from build123d import *

# Parameters (mm, degrees)
BOSS_EXTRUDE1_DEPTH      = 2.5
SKETCH1_R                = 3.11925
SKETCH1_R_2              = 1.61925
BOSS_EXTRUDE2_DEPTH      = 2.5
SKETCH12_R               = 1.61925
CUT_EXTRUDE2_DEPTH       = 3.5
SKETCH15_R               = 3
BOSS_EXTRUDE6_DEPTH      = 2.5
SKETCH13_R               = 1.5
CUT_EXTRUDE5_DEPTH       = 3.5
CUT_EXTRUDE5_DEPTH_BACK  = 3.5
SKETCH16_R               = 3.25
SKETCH16_R_2             = 3.255054338
BOSS_EXTRUDE7_DEPTH      = 2.5
SKETCH17_R               = 1.75
SKETCH17_R_2             = 1.755054338
CUT_EXTRUDE6_DEPTH       = 1
CUT_EXTRUDE6_DEPTH_BACK  = 6
SKETCH24_R               = 1.534588162
SKETCH24_R_2             = 1.539679215
SKETCH24_R_3             = 1.53510928
SKETCH24_R_4             = 1.507254119
SKETCH24_R_5             = 1.501766116
SKETCH24_R_6             = 1.506723366
CUT_EXTRUDE7_DEPTH       = 3.5
CUT_EXTRUDE7_DEPTH_BACK  = 3.5
BOSS_EXTRUDE8_DEPTH      = 23
SKETCH28_W               = 1.910572049
SKETCH28_H               = 15
SKETCH28_W_2             = 2.161085764
CUT_EXTRUDE9_DEPTH       = 3.5
SKETCH30_W               = 30
SKETCH30_H               = 12
SKETCH30_W_2             = 8.543214141
SKETCH30_H_2             = 45.874985667
SKETCH30_H_3             = 29.216310988
SKETCH30_W_3             = 26.664834195
SKETCH30_H_4             = 26.922465443
SKETCH30_W_4             = 17.818641616
SKETCH30_H_5             = 15.402052611
SKETCH30_W_5             = 8.591934673
SKETCH30_H_6             = 73.671406809
CUT_EXTRUDE11_DEPTH      = 3.5
SKETCH29_R               = 12.3
CUT_EXTRUDE12_DEPTH      = 66.426944419
CUT_EXTRUDE12_DEPTH_BACK = 50.584496916
SKETCH31_R               = 1.5
CUT_EXTRUDE13_DEPTH      = 19.369261936
CUT_EXTRUDE13_DEPTH_BACK = 3.5
CUT_EXTRUDE14_DEPTH      = 12


with BuildPart() as part:
    # Sketch2 → Boss-Extrude1 (new body)
    with BuildSketch(Plane(origin=(0, -17.332299444, 0), x_dir=(-1, 0, 0), z_dir=(0, -1, 0))):
        Polygon((125.241603418, -58.531029956), (125.241603418, 41.468970044), (125.241603418, 48.975336237), (115.668802349, 48.975336237), (115.668802349, 41.468970044), (53.135946408, 41.468970044), (53.135946408, 48.975336237), (43.168799778, 48.975336237), (43.168799778, 41.468970044), (-19.254443916, 41.468970044), (-19.254443916, 48.975336237), (-29.674557938, 48.975336237), (-29.674557938, 41.234228149), (-53.610322333, 9.147791006), (-53.610322333, -26.975248892), (-29.352965282, -57.102703243), (-29.352965282, -66.036105098), (-19.352967368, -66.036105098), (-19.352967368, -58.531029956), (43.147035426, -58.531029956), (43.147035426, -66.036105098), (53.147035202, -66.036105098), (53.147035202, -58.531029956), (115.647037996, -58.531029956), (115.647037996, -66.036105098), (125.241603418, -66.036105098), align=None)
    extrude(amount=-BOSS_EXTRUDE1_DEPTH)

    # Sketch1 → Boss-Extrude2 (add)
    with BuildSketch(Plane(origin=(-134.962394185, -12.332299444, 36.871029956), x_dir=(1, 0, 0), z_dir=(0, 1, 0))):
        with Locations((14.01445, 2.71145)):
            Circle(SKETCH1_R)
        with Locations((14.01445, 2.71145)):
            Circle(SKETCH1_R_2, mode=Mode.SUBTRACT)
        with Locations((65.94475, 7.46125)):
            Circle(SKETCH1_R)
        with Locations((65.94475, 7.46125)):
            Circle(SKETCH1_R_2, mode=Mode.SUBTRACT)
        with Locations((65.94475, 35.38855)):
            Circle(SKETCH1_R)
        with Locations((65.94475, 35.38855)):
            Circle(SKETCH1_R_2, mode=Mode.SUBTRACT)
        with Locations((15.15745, 50.62855)):
            Circle(SKETCH1_R)
        with Locations((15.15745, 50.62855)):
            Circle(SKETCH1_R_2, mode=Mode.SUBTRACT)
    extrude(amount=-BOSS_EXTRUDE2_DEPTH)

    # Sketch12 → Cut-Extrude2 (cut, through all)
    with BuildSketch(Plane(origin=(0, -14.832299444, 0), x_dir=(1, 0, 0), z_dir=(0, 1, 0))):
        with Locations((-119.804944185, 13.757520044)):
            Circle(SKETCH12_R)
        with Locations((-69.017644185, -1.482479956)):
            Circle(SKETCH12_R)
        with Locations((-69.017644185, -29.409779956)):
            Circle(SKETCH12_R)
        with Locations((-120.947944185, -34.159579956)):
            Circle(SKETCH12_R)
    extrude(amount=-CUT_EXTRUDE2_DEPTH, mode=Mode.SUBTRACT)

    # Sketch15 → Boss-Extrude6 (add)
    with BuildSketch(Plane(origin=(0, -14.832299444, 0), x_dir=(1, 0, 0), z_dir=(0, 1, 0))):
        with Locations((-46.620694306, -50.539968272)):
            Circle(SKETCH15_R)
        with Locations((-46.620694306, -13.022091641)):
            Circle(SKETCH15_R)
        with Locations((-9.102817675, -50.539968272)):
            Circle(SKETCH15_R)
        with Locations((-9.102817675, -13.022091641)):
            Circle(SKETCH15_R)
    extrude(amount=BOSS_EXTRUDE6_DEPTH)

    # Sketch13 → Cut-Extrude5 (cut, two sides)
    with BuildSketch(Plane(origin=(0, -14.832299444, 0), x_dir=(1, 0, 0), z_dir=(0, 1, 0))) as cut_extrude5_sk:
        with Locations((-46.620694306, -13.022091641)):
            Circle(SKETCH13_R)
        with Locations((-9.102817675, -13.022091641)):
            Circle(SKETCH13_R)
        with Locations((-46.620694306, -50.539968272)):
            Circle(SKETCH13_R)
        with Locations((-9.102817675, -50.539968272)):
            Circle(SKETCH13_R)
    extrude(amount=CUT_EXTRUDE5_DEPTH, mode=Mode.SUBTRACT)
    extrude(cut_extrude5_sk.sketch, amount=-CUT_EXTRUDE5_DEPTH_BACK, mode=Mode.SUBTRACT)

    # Sketch16 → Boss-Extrude7 (add)
    with BuildSketch(Plane(origin=(0, -14.832299444, 0), x_dir=(1, 0, 0), z_dir=(0, 1, 0))):
        with Locations((-11.732899179, 28.299312351)):
            Circle(SKETCH16_R)
        with Locations((-12.172959949, 5.303522595)):
            Circle(SKETCH16_R_2)
        with Locations((-47.166553056, 5.973180288)):
            Circle(SKETCH16_R_2)
        with Locations((-46.726492287, 28.968970044)):
            Circle(SKETCH16_R)
    extrude(amount=BOSS_EXTRUDE7_DEPTH)

    # Sketch17 → Cut-Extrude6 (cut, two sides)
    with BuildSketch(Plane(origin=(0, -12.332299444, 0), x_dir=(1, 0, 0), z_dir=(0, 1, 0))) as cut_extrude6_sk:
        with Locations((-46.726492287, 28.968970044)):
            Circle(SKETCH17_R)
        with Locations((-47.166553056, 5.973180288)):
            Circle(SKETCH17_R_2)
        with Locations((-12.172959949, 5.303522595)):
            Circle(SKETCH17_R_2)
        with Locations((-11.732899179, 28.299312351)):
            Circle(SKETCH17_R)
    extrude(amount=CUT_EXTRUDE6_DEPTH, mode=Mode.SUBTRACT)
    extrude(cut_extrude6_sk.sketch, amount=-CUT_EXTRUDE6_DEPTH_BACK, mode=Mode.SUBTRACT)

    # Sketch24 → Cut-Extrude7 (cut, two sides)
    with BuildSketch(Plane(origin=(0, -14.832299444, 0), x_dir=(1, 0, 0), z_dir=(0, 1, 0))) as cut_extrude7_sk:
        with Locations((-120.631514326, 43.936289371)):
            Circle(SKETCH24_R)
        with Locations((-48.193182725, 43.936289371)):
            Circle(SKETCH24_R_2)
        with Locations((24.374871647, 43.936289371)):
            Circle(SKETCH24_R_3)
        with Locations((24.374871647, -61.035755979)):
            Circle(SKETCH24_R_4)
        with Locations((-48.193182725, -61.035755979)):
            Circle(SKETCH24_R_5)
        with Locations((-120.631514326, -61.035755979)):
            Circle(SKETCH24_R_6)
    extrude(amount=CUT_EXTRUDE7_DEPTH, mode=Mode.SUBTRACT)
    extrude(cut_extrude7_sk.sketch, amount=-CUT_EXTRUDE7_DEPTH_BACK, mode=Mode.SUBTRACT)

    # Sketch25 → Boss-Extrude8 (add)
    with BuildSketch(Plane(origin=(0, -14.832299444, 0), x_dir=(1, 0, 0), z_dir=(0, 1, 0))):
        Polygon((25.524416428, 37.468970044), (32.483356263, 37.468970044), (42.544257405, 23.982102995), (42.544257405, -40.719218001), (31.423568275, -54.531029956), (25.524416428, -54.531029956), align=None)
    extrude(amount=BOSS_EXTRUDE8_DEPTH)

    # Sketch28 → Cut-Extrude9 (cut, through all)
    with BuildSketch(Plane(origin=(0, -14.832299444, 0), x_dir=(1, 0, 0), z_dir=(0, 1, 0))):
        with Locations((21.640674678, -25.829400353)):
            Rectangle(SKETCH28_W, SKETCH28_H)
        with Locations((21.640674678, 8.33851306)):
            Rectangle(SKETCH28_W, SKETCH28_H)
        with Locations((48.076503584, -25.829400353)):
            Rectangle(SKETCH28_W_2, SKETCH28_H)
        with Locations((48.076503584, 8.33851306)):
            Rectangle(SKETCH28_W_2, SKETCH28_H)
    extrude(amount=-CUT_EXTRUDE9_DEPTH, mode=Mode.SUBTRACT)

    # Sketch30 → Cut-Extrude11 (cut, through all)
    with BuildSketch(Plane(origin=(0, -14.832299444, 0), x_dir=(1, 0, 0), z_dir=(0, 1, 0))):
        with Locations((-95.241603418, -42.531029956)):
            Rectangle(SKETCH30_W, SKETCH30_H)
        with Locations((-95.241603418, 25.468970044)):
            Rectangle(SKETCH30_W, SKETCH30_H)
        with Locations((-57.539223691, -11.460765675)):
            Rectangle(SKETCH30_W_2, SKETCH30_H_2)
        with Locations((-95.241603418, -8.701691218)):
            Rectangle(SKETCH30_W, SKETCH30_H_3)
        with Locations((-28.677773335, -31.68039269)):
            Rectangle(SKETCH30_W_3, SKETCH30_H_4)
        with Locations((-29.547493126, 17.632663699)):
            Rectangle(SKETCH30_W_4, SKETCH30_H_5)
        with Locations((4.295967337, -8.305922008)):
            Rectangle(SKETCH30_W_5, SKETCH30_H_6)
    extrude(amount=-CUT_EXTRUDE11_DEPTH, mode=Mode.SUBTRACT)

    # Sketch29 → Cut-Extrude12 (cut, two sides)
    with BuildSketch(Plane(origin=(0, 0, 16.451608182), x_dir=(-1, 0, 0), z_dir=(0, 0, -1))) as cut_extrude12_sk:
        with Locations((-34.72344809, 11.701998712)):
            Circle(SKETCH29_R)
    extrude(amount=CUT_EXTRUDE12_DEPTH, mode=Mode.SUBTRACT)
    extrude(cut_extrude12_sk.sketch, amount=-CUT_EXTRUDE12_DEPTH_BACK, mode=Mode.SUBTRACT)

    # Sketch31 → Cut-Extrude13 (cut, two sides)
    with BuildSketch(Plane(origin=(0, -14.832299444, 0), x_dir=(1, 0, 0), z_dir=(0, 1, 0))) as cut_extrude13_sk:
        with Locations((50.610322333, -12.329400353)):
            Circle(SKETCH31_R)
        with Locations((50.610322333, -5.16148694)):
            Circle(SKETCH31_R)
    extrude(amount=CUT_EXTRUDE13_DEPTH, mode=Mode.SUBTRACT)
    extrude(cut_extrude13_sk.sketch, amount=-CUT_EXTRUDE13_DEPTH_BACK, mode=Mode.SUBTRACT)

    # Sketch32 → Cut-Extrude14 (cut)
    with BuildSketch(Plane.XZ.offset(17.332299444)):
        Polygon((30.524416428, 47.675089459), (30.524416428, -31.732854607), (37.544257405, -22.322597948), (37.544257405, 38.956499954), align=None)
    extrude(amount=-CUT_EXTRUDE14_DEPTH, mode=Mode.SUBTRACT)


solid = part.part
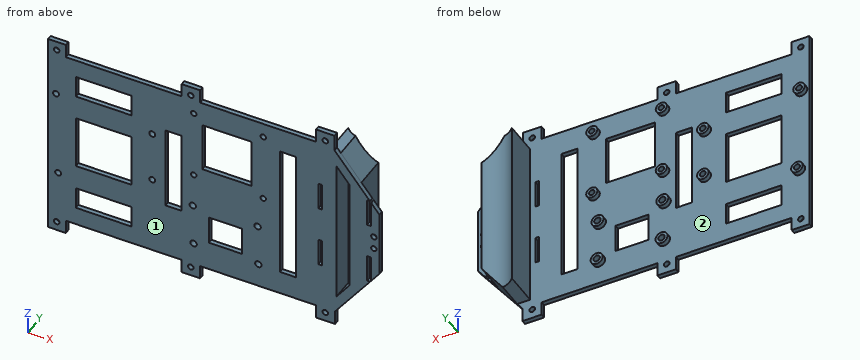
Can you work these out from the model? Positions are in its coordinate system, mm. Face numbers are marked on the shaded views. Round coordinates to 2 decimals unless told otherwise and drop trailing zeros. Loops run counter-clockwise (first coordinate to the right, second up) from the corner with the lowest first, then second, coordinate; pieces in that order, holes last. Notation, with made-up numbers: (-6.5, -16.75) - (1.5, -16.75) arc R16 ccw to (1.5, 6.25) - close; hole circle Ø10 at (72, 2.25). An arc over 180 degrees is marked (long way). Use CSV: the item, a comma, the result in double quotes. Start each with the question number.
1) Please list where these lines run through material, in increasing order: probe 1 along X at (y, z) = (-15, 15); probe 2 along X at (y, z) = (-12, 24.5); probe 3 along Y at (x, z) = (-21, -9). Write a range as [from, to].
2) If we section it at C-C on x = -83.5: Write out the boundary of the cut face in (y, z), plus the area to 3 significant figures.
3) For pin 1 Ø5 at (x, z) = (24.37, 61.04) entering from -Y; pin 2 Ø3 at (y, z) = (-1.5, 2) entering from +X; pin 3 Ø1 at (x, z) = (-7.5, -18.5) entering from +Y; pin 4 Ø10 at (x, z) = (-7, -22.5) entering from +Y, each with a flat end and sliding along its axis, tell me the tip position at first contact or that it passes through.
4) If we section it at B-B on y = -8: Write out the boundary of the cut face in (x, z), plus the area to 3 significant figures.
5) If we section it at A-A on x = -17.5: Write out the boundary of the cut face in (y, z), plus the area to 3 significant figures.
6) We'd pull the mould along X, two halves only. Please class the marked faces 1 and 2: released by +X, released by -X, zero draft, split by the parting line, or undercut.
Geometry results:
1,probe 1,"x = [-125.24, -110.24], [-80.24, -61.81], [-53.27, 0], [8.59, 30.52], [37.54, 53.61]"
1,probe 2,"x = [25.52, 30.52], [37.54, 42.54]"
1,probe 3,"y = [-17.33, -14.83]"
2,outline,"(-17.33, -41.47) - (-14.83, -41.47) - (-14.83, -31.47) - (-17.33, -31.47) - close; (-17.33, -19.47) - (-14.83, -19.47) - (-14.83, -5.91) - (-17.33, -5.91) - close; (-17.33, 23.31) - (-14.83, 23.31) - (-14.83, 36.53) - (-17.33, 36.53) - close; (-17.33, 48.53) - (-14.83, 48.53) - (-14.83, 58.53) - (-17.33, 58.53) - close"
2,area,"117 mm2"
3,pin 1,"stops at y = -17.33"
3,pin 2,"stops at x = 42.54"
3,pin 3,"stops at y = -14.83"
3,pin 4,"stops at y = -12.33"
4,outline,"(25.52, -37.47) - (32.48, -37.47) - (42.54, -23.98) - (42.54, 40.72) - (31.42, 54.53) - (25.52, 54.53) - close; hole (30.52, -31.73) - (37.54, -22.32) - (37.54, 38.96) - (30.52, 47.68) - close"
4,area,"927 mm2"
5,outline,"(-17.33, -41.47) - (-14.83, -41.47) - (-14.83, 18.22) - (-17.33, 18.22) - close; (-17.33, 45.14) - (-14.83, 45.14) - (-14.83, 58.53) - (-17.33, 58.53) - close"
5,area,"183 mm2"
6,face 1,"zero draft"
6,face 2,"undercut"
